```python
from build123d import *

# Parameters (mm, degrees)
SKETCH_1_W          = 50
SKETCH_1_H          = 30
EXTRUDE_1_DEPTH     = 25
SKETCH_2_R          = 5
EXTRUDE_2_DEPTH     = 1
SKETCH_3_R          = 4
EXTRUDE_3_DEPTH     = 15
SKETCH_6_W          = 125.650571392
SKETCH_6_H          = 76.942116616
SKETCH_6_W_2        = 31.088556847
SKETCH_6_H_2        = 20
CUT_EXTRUDE_1_DEPTH = 39.405728739
SKETCH_7_W          = 12.5
SKETCH_7_H          = 20
CUT_EXTRUDE_2_DEPTH = 53.416584845
SKETCH_8_R          = 7.5
EXTRUDE_5_DEPTH     = 20
SKETCH_9_W          = 1.5
SKETCH_9_H          = 0.5
EXTRUDE_6_DEPTH     = 2
SKETCH_10_R         = 0.3
CUT_EXTRUDE_3_DEPTH = 2
FILLET_1_R          = 0.5
CUT_EXTRUDE_START   = -7
CUT_EXTRUDE_4_DEPTH = 7
SKETCH_12_R         = 1
CUT_EXTRUDE_5_DEPTH = 54.572073189


with BuildPart() as part:
    # 草图1 → 凸台-拉伸1 (new body)
    with BuildSketch(Plane.XY):
        Rectangle(SKETCH_1_W, SKETCH_1_H)
    extrude(amount=EXTRUDE_1_DEPTH)

    # 草图2 → 凸台-拉伸2 (add)
    with BuildSketch(Plane.XY.offset(25)):
        with Locations((-15, 0)):
            Circle(SKETCH_2_R)
    extrude(amount=EXTRUDE_2_DEPTH)

    # 草图3 → 凸台-拉伸3 (add)
    with BuildSketch(Plane.XY.offset(26)):
        with Locations((-15, 0)):
            Circle(SKETCH_3_R)
    extrude(amount=EXTRUDE_3_DEPTH)

    # 草图6 → 切除-拉伸1 (cut, through all)
    with BuildSketch(Plane.XY.offset(25)):
        with Locations((-32.975192835, 18.238730024)):
            Rectangle(SKETCH_6_W, SKETCH_6_H)
        with Locations((-9.455721577, 0)):
            Rectangle(SKETCH_6_W_2, SKETCH_6_H_2, mode=Mode.SUBTRACT)
    extrude(amount=-CUT_EXTRUDE_1_DEPTH, mode=Mode.SUBTRACT)

    # 草图7 → 切除-拉伸2 (cut, through all)
    with BuildSketch(Plane(origin=(6.088556847, 0, 0), x_dir=(0, 0, -1), z_dir=(1, 0, 0))):
        with Locations((-6.25, 0)):
            Rectangle(SKETCH_7_W, SKETCH_7_H)
    extrude(amount=-CUT_EXTRUDE_2_DEPTH, mode=Mode.SUBTRACT)

    # 草图8 → 凸台-拉伸5 (add)
    with BuildSketch(Plane(origin=(6.088556847, 0, 0), x_dir=(0, 0, -1), z_dir=(1, 0, 0))):
        with Locations(Location((-18.75, 0, 0), (0, 0, 146.442690238))):
            Circle(SKETCH_8_R)
    extrude(amount=EXTRUDE_5_DEPTH)

    # 草图9 → 凸台-拉伸6 (add)
    with BuildSketch(Plane(origin=(26.088556847, 0, 0), x_dir=(0, 0, -1), z_dir=(1, 0, 0))):
        with Locations((-23.75, 0)):
            Rectangle(SKETCH_9_W, SKETCH_9_H)
        with Locations((-13.75, 0)):
            Rectangle(SKETCH_9_W, SKETCH_9_H)
    extrude(amount=EXTRUDE_6_DEPTH)

    # 草图10 → 切除-拉伸3 (cut)
    with BuildSketch(Plane.XZ.offset(0.25)):
        with Locations(Location((27.088556847, 23.75, 0), (0, 0, 270))):
            Circle(SKETCH_10_R)
        with Locations(Location((27.088556847, 13.75, 0), (0, 0, 270))):
            Circle(SKETCH_10_R)
    extrude(amount=-CUT_EXTRUDE_3_DEPTH, mode=Mode.SUBTRACT)

    # 圆角1
    # the kernel refuses this fillet: 0.5 mm, written as the material it takes off along each edge
    with BuildSketch(Plane(origin=(-24.5, -9.5, 24.5), x_dir=(0, 0, 1), z_dir=(-1, 0, 0))) as fillet_1_piece_1_section:
        Polygon((0, 0), (FILLET_1_R * 1.02, 0), (FILLET_1_R * 1.02, -FILLET_1_R * 1.02), (0, -FILLET_1_R * 1.02), align=None)
    fillet_1_piece_1 = extrude(amount=FILLET_1_R * 1.02, mode=Mode.PRIVATE)
    fillet_1_piece_1 = fillet_1_piece_1 - Plane(origin=(-24.5, -9.5, 24.5), x_dir=(0, 0.7071067811865475, -0.7071067811865475), z_dir=(-1, 0, 0)) * Sphere(FILLET_1_R, mode=Mode.PRIVATE)
    add(fillet_1_piece_1, mode=Mode.SUBTRACT)
    with BuildSketch(Plane(origin=(-24.5, 9.5, 24.5), x_dir=(0, 1, 0), z_dir=(-1, 0, 0))) as fillet_1_piece_2_section:
        Polygon((0, 0), (FILLET_1_R * 1.02, 0), (FILLET_1_R * 1.02, -FILLET_1_R * 1.02), (0, -FILLET_1_R * 1.02), align=None)
    fillet_1_piece_2 = extrude(amount=FILLET_1_R * 1.02, mode=Mode.PRIVATE)
    fillet_1_piece_2 = fillet_1_piece_2 - Plane(origin=(-24.5, 9.5, 24.5), x_dir=(0, -0.7071067811865475, -0.7071067811865475), z_dir=(-1, 0, 0)) * Sphere(FILLET_1_R, mode=Mode.PRIVATE)
    add(fillet_1_piece_2, mode=Mode.SUBTRACT)
    with BuildSketch(Plane(origin=(5.588556847, 9.5, 24.5), x_dir=(0, 0, 1), z_dir=(0, 1, 0))) as fillet_1_piece_3_section:
        Polygon((0, 0), (FILLET_1_R * 1.02, 0), (FILLET_1_R * 1.02, FILLET_1_R * 1.02), (0, FILLET_1_R * 1.02), align=None)
    fillet_1_piece_3 = extrude(amount=FILLET_1_R * 1.02, mode=Mode.PRIVATE)
    fillet_1_piece_3 = fillet_1_piece_3 - Plane(origin=(5.588556847, 9.5, 24.5), x_dir=(-0.7071067811865475, 0, -0.7071067811865475), z_dir=(0, 1, 0)) * Sphere(FILLET_1_R, mode=Mode.PRIVATE)
    add(fillet_1_piece_3, mode=Mode.SUBTRACT)
    with BuildSketch(Plane(origin=(5.588556847, -9.5, 24.5), x_dir=(0, -1, 0), z_dir=(0, 0, 1))) as fillet_1_piece_4_section:
        Polygon((0, 0), (FILLET_1_R * 1.02, 0), (FILLET_1_R * 1.02, FILLET_1_R * 1.02), (0, FILLET_1_R * 1.02), align=None)
    fillet_1_piece_4 = extrude(amount=FILLET_1_R * 1.02, mode=Mode.PRIVATE)
    fillet_1_piece_4 = fillet_1_piece_4 - Plane(origin=(5.588556847, -9.5, 24.5), x_dir=(-0.7071067811865475, 0.7071067811865476, 0), z_dir=(0, 0, 1)) * Sphere(FILLET_1_R, mode=Mode.PRIVATE)
    add(fillet_1_piece_4, mode=Mode.SUBTRACT)
    with BuildSketch(Plane(origin=(-24.5, -9.5, 13), x_dir=(0, 0, -1), z_dir=(-1, 0, 0))) as fillet_1_piece_5_section:
        Polygon((0, 0), (FILLET_1_R * 1.02, 0), (FILLET_1_R * 1.02, FILLET_1_R * 1.02), (0, FILLET_1_R * 1.02), align=None)
    fillet_1_piece_5 = extrude(amount=FILLET_1_R * 1.02, mode=Mode.PRIVATE)
    fillet_1_piece_5 = fillet_1_piece_5 - Plane(origin=(-24.5, -9.5, 13), x_dir=(0, 0.7071067811865475, 0.7071067811865475), z_dir=(-1, 0, 0)) * Sphere(FILLET_1_R, mode=Mode.PRIVATE)
    add(fillet_1_piece_5, mode=Mode.SUBTRACT)
    with BuildSketch(Plane(origin=(5.588556847, -9.5, 13), x_dir=(0, -1, 0), z_dir=(0, 0, -1))) as fillet_1_piece_6_section:
        Polygon((0, 0), (FILLET_1_R * 1.02, 0), (FILLET_1_R * 1.02, -FILLET_1_R * 1.02), (0, -FILLET_1_R * 1.02), align=None)
    fillet_1_piece_6 = extrude(amount=FILLET_1_R * 1.02, mode=Mode.PRIVATE)
    fillet_1_piece_6 = fillet_1_piece_6 - Plane(origin=(5.588556847, -9.5, 13), x_dir=(-0.7071067811865475, 0.7071067811865476, 0), z_dir=(0, 0, -1)) * Sphere(FILLET_1_R, mode=Mode.PRIVATE)
    add(fillet_1_piece_6, mode=Mode.SUBTRACT)
    with BuildSketch(Plane(origin=(5.588556847, 9.5, 13), x_dir=(0, 1, 0), z_dir=(0, 0, -1))) as fillet_1_piece_7_section:
        Polygon((0, 0), (FILLET_1_R * 1.02, 0), (FILLET_1_R * 1.02, FILLET_1_R * 1.02), (0, FILLET_1_R * 1.02), align=None)
    fillet_1_piece_7 = extrude(amount=FILLET_1_R * 1.02, mode=Mode.PRIVATE)
    fillet_1_piece_7 = fillet_1_piece_7 - Plane(origin=(5.588556847, 9.5, 13), x_dir=(-0.7071067811865475, -0.7071067811865476, 0), z_dir=(0, 0, -1)) * Sphere(FILLET_1_R, mode=Mode.PRIVATE)
    add(fillet_1_piece_7, mode=Mode.SUBTRACT)
    with BuildSketch(Plane(origin=(-24.5, 9.5, 13), x_dir=(0, 0, -1), z_dir=(-1, 0, 0))) as fillet_1_piece_8_section:
        Polygon((0, 0), (FILLET_1_R * 1.02, 0), (FILLET_1_R * 1.02, -FILLET_1_R * 1.02), (0, -FILLET_1_R * 1.02), align=None)
    fillet_1_piece_8 = extrude(amount=FILLET_1_R * 1.02, mode=Mode.PRIVATE)
    fillet_1_piece_8 = fillet_1_piece_8 - Plane(origin=(-24.5, 9.5, 13), x_dir=(0, -0.7071067811865475, 0.7071067811865475), z_dir=(-1, 0, 0)) * Sphere(FILLET_1_R, mode=Mode.PRIVATE)
    add(fillet_1_piece_8, mode=Mode.SUBTRACT)
    with BuildSketch(Plane(origin=(-25, -9.5, 25), x_dir=(0, 0, -1), z_dir=(0, 1, 0)), Plane(origin=(-25, 9.5, 12.5), x_dir=(0, 0, 1), z_dir=(0, -1, 0))) as fillet_1_piece_9:
        with BuildLine():
            CenterArc((FILLET_1_R, -FILLET_1_R), FILLET_1_R, 90, 90)
            Line((0, -FILLET_1_R), (0, 0))
            Line((0, 0), (FILLET_1_R, 0))
        make_face()
    extrude(amount=19, mode=Mode.SUBTRACT)
    with BuildSketch(Plane(origin=(-24.5, 10, 25), x_dir=(0, 0, -1), z_dir=(1, 0, 0)), Plane(origin=(5.588556847, -10, 12.5), x_dir=(0, 1, 0), z_dir=(-1, 0, 0))) as fillet_1_piece_10:
        with BuildLine():
            CenterArc((FILLET_1_R, -FILLET_1_R), FILLET_1_R, 90, 90)
            Line((0, -FILLET_1_R), (0, 0))
            Line((0, 0), (FILLET_1_R, 0))
        make_face()
    extrude(amount=30.088556847, mode=Mode.SUBTRACT)
    with BuildSketch(Plane(origin=(6.088556847, -2.895780988, 25), x_dir=(-1, 0, 0), z_dir=(0, -1, 0))) as fillet_1_piece_11_section:
        with BuildLine():
            CenterArc((FILLET_1_R, FILLET_1_R), FILLET_1_R, 180, 90)
            Line((0, FILLET_1_R), (0, 0))
            Line((0, 0), (FILLET_1_R, 0))
        make_face()
    fillet_1_piece_11 = extrude(amount=6.604219012, mode=Mode.PRIVATE)
    fillet_1_piece_11 = fillet_1_piece_11 - Plane(origin=(5.975472157, 0, 18.75), x_dir=(0, 0.5527707983937196, 0.8333333333325685), z_dir=(-1, 0, 0)) * Cylinder(7.5, 16, mode=Mode.PRIVATE)
    add(fillet_1_piece_11, mode=Mode.SUBTRACT)
    with BuildSketch(Plane(origin=(5.588556847, -10, 25), x_dir=(0, 1, 0), z_dir=(-1, 0, 0)), Plane(origin=(5.588556847, 10, 12.5), x_dir=(0, -1, 0), z_dir=(-1, 0, 0))) as fillet_1_piece_12:
        with BuildLine():
            CenterArc((FILLET_1_R, FILLET_1_R), FILLET_1_R, 180, 90)
            Line((0, FILLET_1_R), (0, 0))
            Line((0, 0), (FILLET_1_R, 0))
        make_face()
    extrude(amount=30.088556847, mode=Mode.SUBTRACT)
    with BuildSketch(Plane(origin=(-25, -10, 24.5), x_dir=(0, 1, 0), z_dir=(0, 0, -1)), Plane(origin=(6.088556847, -10, 24.5), x_dir=(-1, 0, 0), z_dir=(0, 0, -1))) as fillet_1_piece_13:
        with BuildLine():
            CenterArc((FILLET_1_R, FILLET_1_R), FILLET_1_R, 180, 90)
            Line((0, FILLET_1_R), (0, 0))
            Line((0, 0), (FILLET_1_R, 0))
        make_face()
    extrude(amount=11.5, mode=Mode.SUBTRACT)
    with BuildSketch(Plane(origin=(6.088556847, 10, 24.5), x_dir=(-1, 0, 0), z_dir=(0, 0, -1)), Plane(origin=(-25, 10, 24.5), x_dir=(0, -1, 0), z_dir=(0, 0, -1))) as fillet_1_piece_14:
        with BuildLine():
            CenterArc((FILLET_1_R, -FILLET_1_R), FILLET_1_R, 90, 90)
            Line((0, -FILLET_1_R), (0, 0))
            Line((0, 0), (FILLET_1_R, 0))
        make_face()
    extrude(amount=11.5, mode=Mode.SUBTRACT)
    with BuildSketch(Plane(origin=(6.088556847, 2.895780988, 12.5), x_dir=(-1, 0, 0), z_dir=(0, 1, 0))) as fillet_1_piece_15_section:
        with BuildLine():
            CenterArc((FILLET_1_R, FILLET_1_R), FILLET_1_R, 180, 90)
            Line((0, FILLET_1_R), (0, 0))
            Line((0, 0), (FILLET_1_R, 0))
        make_face()
    fillet_1_piece_15 = extrude(amount=6.604219012, mode=Mode.PRIVATE)
    fillet_1_piece_15 = fillet_1_piece_15 - Plane(origin=(5.975472139, 0, 18.75), x_dir=(0, 0.5527707983937196, 0.8333333333325685), z_dir=(-1, 0, 0)) * Cylinder(7.5, 16, mode=Mode.PRIVATE)
    add(fillet_1_piece_15, mode=Mode.SUBTRACT)
    with BuildSketch(Plane(origin=(6.088556847, -9.5, 12.5), x_dir=(-1, 0, 0), z_dir=(0, 1, 0))) as fillet_1_piece_16_section:
        with BuildLine():
            CenterArc((FILLET_1_R, FILLET_1_R), FILLET_1_R, 180, 90)
            Line((0, FILLET_1_R), (0, 0))
            Line((0, 0), (FILLET_1_R, 0))
        make_face()
    fillet_1_piece_16 = extrude(amount=6.604219012, mode=Mode.PRIVATE)
    fillet_1_piece_16 = fillet_1_piece_16 - Plane(origin=(5.97547253, 0, 18.75), x_dir=(0, 0.5527707983937196, 0.8333333333325685), z_dir=(-1, 0, 0)) * Cylinder(7.5, 16, mode=Mode.PRIVATE)
    add(fillet_1_piece_16, mode=Mode.SUBTRACT)
    with BuildSketch(Plane(origin=(6.088556847, 9.5, 25), x_dir=(-1, 0, 0), z_dir=(0, -1, 0))) as fillet_1_piece_17_section:
        with BuildLine():
            CenterArc((FILLET_1_R, FILLET_1_R), FILLET_1_R, 180, 90)
            Line((0, FILLET_1_R), (0, 0))
            Line((0, 0), (FILLET_1_R, 0))
        make_face()
    fillet_1_piece_17 = extrude(amount=6.604219012, mode=Mode.PRIVATE)
    fillet_1_piece_17 = fillet_1_piece_17 - Plane(origin=(5.975472488, 0, 18.75), x_dir=(0, 0.5527707983937196, 0.8333333333325685), z_dir=(-1, 0, 0)) * Cylinder(7.5, 16, mode=Mode.PRIVATE)
    add(fillet_1_piece_17, mode=Mode.SUBTRACT)

    # 草图11 → 切除-拉伸4 (cut)
    with BuildSketch(Plane.XY.offset(41).offset(CUT_EXTRUDE_START)):
        with BuildLine():
            Line((-12.989168341, 3.457825334), (-12.989168341, -3.457825334))
            ThreePointArc((-12.989168341, -3.457825334), (-11, 0), (-12.989168341, 3.457825334))
        make_face()
    extrude(amount=CUT_EXTRUDE_4_DEPTH, mode=Mode.SUBTRACT)

    # 草图12 → 切除-拉伸5 (cut, through all)
    with BuildSketch(Plane.XZ.offset(10)):
        with Locations((-22.5, 22.5)):
            Circle(SKETCH_12_R)
        with Locations((3.588556847, 22.5)):
            Circle(SKETCH_12_R)
        with Locations((-22.5, 15)):
            Circle(SKETCH_12_R)
        with Locations((3.588556847, 15)):
            Circle(SKETCH_12_R)
    extrude(amount=-CUT_EXTRUDE_5_DEPTH, mode=Mode.SUBTRACT)


solid = part.part
```
CAD build for the part. Positions are in the model's coordinates, mm. A direction names the side the tool comes from. Round coordinates to 2 decimals unless told otherwise and drop trailing zeros. Write each loop counter-clockwise with the first axis right and the second up, starting at its lowest first coordinate (ties: lowest second). Pieces come first, ordered by that corner, then holes.
Item 1: Band-saw the part on C-C on x = -15. Write the cut outline in (y, z).
Filled in:
outline: (-10, 13) arc R0.5 ccw to (-9.5, 12.5) - (9.5, 12.5) arc R0.5 ccw to (10, 13) - (10, 24.5) arc R0.5 ccw to (9.5, 25) - (5, 25) - (5, 26) - (4, 26) - (4, 41) - (-4, 41) - (-4, 26) - (-5, 26) - (-5, 25) - (-9.5, 25) arc R0.5 ccw to (-10, 24.5) - close
Item 2: Drop flat-ended pins along their axis: pin 1 Ø3 at (x, z) = (-22.5, 15) entering from +Y; pin 2 Ø5 at (x, y) = (-12.5, 7) entering from +Z; pin 3 Ø0.6 at (x, y) = (27.5, 0) entering from +Z; pin 4 Ø5 at (y, z) = (7.5, 20.5) entering from +X. Give the stop position or say it passes through.
Filled in:
pin 1: stops at y = 10
pin 2: stops at z = 26
pin 3: stops at z = 24.5
pin 4: stops at x = 26.09
Item 3: Band-saw the part on A-A on x = -22.5. Write the cut outline in (y, z).
Filled in:
outline: (-10, 13) arc R0.5 ccw to (-9.5, 12.5) - (9.5, 12.5) arc R0.5 ccw to (10, 13) - (10, 14) - (-10, 14) - close; (-10, 16) - (10, 16) - (10, 21.5) - (-10, 21.5) - close; (-10, 23.5) - (10, 23.5) - (10, 24.5) arc R0.5 ccw to (9.5, 25) - (-9.5, 25) arc R0.5 ccw to (-10, 24.5) - close
Item 4: Tool access for faces 1 (the flat face through (6.089, -8, 19)), 2 (the flat face through (-12.989, 0, 37)), 3 (the flat face through (-9, 0, 12.5)), 4 (the flat face through (6.089, 8, 19)), 5 (the cylindrical face through (-18.2, -2.4, 33.4)): list every direction of +Z, -Z, +X, -X, +Y, -Y with a clear straight run to the whole face (end or side of a thin tool).
Filled in:
face 1: +X, -Y
face 2: +Z, +X, +Y, -Y
face 3: -Z, -X, +Y, -Y
face 4: +X, +Y
face 5: +Z
Item 5: Drill centre lines: L1, parallel to Z at x = -22.5, y = -2.5; L2, parallel to Z at x = -7, y = -7.25; L3, parallel to X at y = 7.5, z = 13.25. Where is each one in solid material? Low to high.
Filled in:
L1: z = 12.5 to 14, 16 to 21.5, 23.5 to 25
L2: z = 12.5 to 25
L3: x = -25 to 6.09
Item 6: Mould opens along Z. For faces 6 (the cylindrical face through (3.372, -0.14, 21.524)), 7 (the cylindrical face through (3.372, -0.14, 14.024)), 8 (the cylindrical face through (-19.995, 0.22, 25.493)), 9 (the flat face through (-12, 0, 34)) say: released by +Z, released by -Z, zero draft, split by the parting line, or undercut.
Filled in:
face 6: undercut
face 7: undercut
face 8: zero draft
face 9: released by +Z
Item 7: Band-saw the part on D-D on z = 29. Write the cut outline in (x, y).
Filled in:
outline: circle Ø8 at (-15, 0)
Item 8: Band-saw the part on B-B on z = 18.75. Write the cut outline in (x, y), then the cut area to 3 significant figures.
Filled in:
outline: (-25, -9.5) arc R0.5 ccw to (-24.5, -10) - (5.59, -10) arc R0.5 ccw to (6.09, -9.5) - (6.09, -7.5) - (26.09, -7.5) - (26.09, 7.5) - (6.09, 7.5) - (6.09, 9.5) arc R0.5 ccw to (5.59, 10) - (-24.5, 10) arc R0.5 ccw to (-25, 9.5) - close
area: 922 mm2
